Source: CAD feature listing. Evaluate the final solid. Frame: model axes, mm. Coordinates: 2 decimals unless noted, no trailing zeros.
```python
from build123d import *

# Parameters (mm, degrees)
EXTRUDE_1_DEPTH              = 8
HOLE_WIZARD_M3_2_D           = 3
HOLE_WIZARD_M5_1_D           = 8
HOLE_WIZARD_M5_1_CBORE_D     = 9.5
HOLE_WIZARD_M5_1_CBORE_DEPTH = 0.9
SKETCH_11_R                  = 1.5
CUT_EXTRUDE_1_DEPTH          = 1
CUT_EXTRUDE_1_DEPTH_BACK     = 9


with BuildPart() as part:
    # 草图1 → 凸台-拉伸1 (new body)
    with BuildSketch(Plane.XY):
        with BuildLine():
            Line((77.5, 10), (-77.5, 10))
            ThreePointArc((-77.5, 10), (-70.428932188, 7.071067812), (-67.5, 0))
            ThreePointArc((-67.5, 0), (-70.428932188, -7.071067812), (-77.5, -10))
            Line((-77.5, -10), (77.5, -10))
            ThreePointArc((77.5, -10), (87.5, 0), (77.5, 10))
        make_face()
        with BuildLine():
            ThreePointArc((-67.5, 0), (-70.428932188, 7.071067812), (-77.5, 10))
            ThreePointArc((-77.5, 10), (-78.000627751, 9.987460731), (-78.5, 9.949874371))
            ThreePointArc((-78.5, 9.949874371), (-87.5, 0), (-78.5, -9.949874371))
            ThreePointArc((-78.5, -9.949874371), (-78.000627751, -9.987460731), (-77.5, -10))
            ThreePointArc((-77.5, -10), (-70.428932188, -7.071067812), (-67.5, 0))
        make_face()
        with BuildLine():
            ThreePointArc((-78.5, -9.949874371), (-87.5, 0), (-78.5, 9.949874371))
            Line((-78.5, 9.949874371), (-103.25, 7.462405778))
            ThreePointArc((-103.25, 7.462405778), (-110, 0), (-103.25, -7.462405778))
            Line((-103.25, -7.462405778), (-78.5, -9.949874371))
        make_face()
    extrude(amount=EXTRUDE_1_DEPTH)

    # M3 螺纹孔2 (through all)
    with Locations(Plane.XY.offset(8)):
        with Locations((-78.5, 0), (-93.5, 0), (-82.5, 0)):
            Hole(HOLE_WIZARD_M3_2_D / 2)

    # M5 六角头螺栓的柱形沉头孔1 (through all)
    with Locations(Plane.XY.offset(8)):
        with Locations((-102.5, 0), (77.5, 0)):
            CounterBoreHole(HOLE_WIZARD_M5_1_D / 2, HOLE_WIZARD_M5_1_CBORE_D / 2, HOLE_WIZARD_M5_1_CBORE_DEPTH)

    # 草图11 → 切除-拉伸1 (cut, two sides)
    with BuildSketch(Plane.XY.offset(8)) as cut_extrude_1_sk:
        with Locations((-52.5, 0)):
            Circle(SKETCH_11_R)
        with Locations((-25.5, 0)):
            Circle(SKETCH_11_R)
        with Locations((1.5, 0)):
            Circle(SKETCH_11_R)
        with Locations((28.5, 0)):
            Circle(SKETCH_11_R)
        with Locations((55.5, 0)):
            Circle(SKETCH_11_R)
    extrude(amount=CUT_EXTRUDE_1_DEPTH, mode=Mode.SUBTRACT)
    extrude(cut_extrude_1_sk.sketch, amount=-CUT_EXTRUDE_1_DEPTH_BACK, mode=Mode.SUBTRACT)


solid = part.part
```
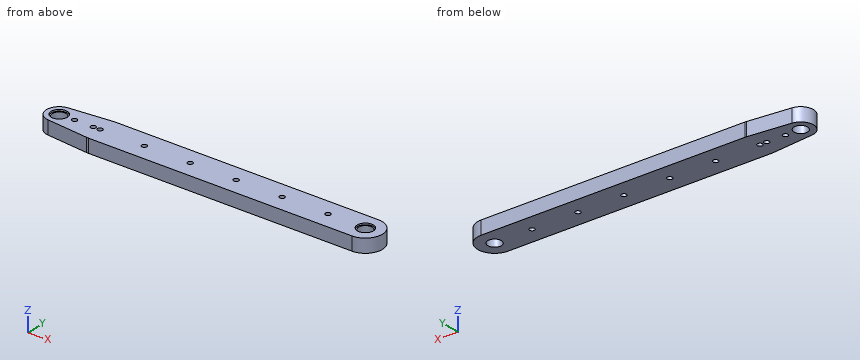
Q1. Pin query (flat end, axial travel): P1, Ø5, axis at x = 55.5, y = 0, coming from the +Z side; P2, Ø5, axis at x = 76.5, y = -0.5, coming from the +Z side. Return the tip coordinate at first contact, or that it passes through.
Solutions:
P1: stops at z = 8
P2: passes through
Q2. Section query A-A on z = 5.5. Give the number of separate pieces and of enclosed holes in the cut face, plus the area to 3 significant figures.
Solutions:
separate pieces: 1
enclosed holes: 10
area: 3,630 mm2
Q3. Material intervals for line 1 along Y through (x, z) = (55.5, 3.5); line 2 along X through (y, z) = (-1.75, 0.5); line 3 along Y through (x, z) = (77.5, 2), sorted ascending.
Solutions:
line 1: y = -10 to -1.5, 1.5 to 10
line 2: x = -109.79 to -106.1, -98.9 to 73.9, 81.1 to 87.35
line 3: y = -10 to -4, 4 to 10
